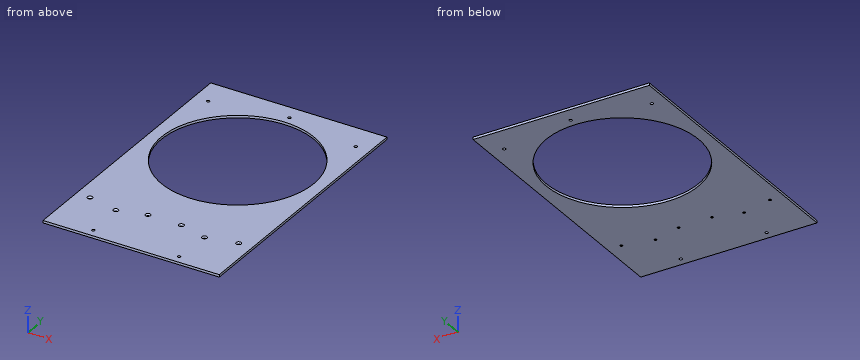
```python
from build123d import *

# Parameters (mm, degrees)
SKETCH1_W                                     = 469.9
SKETCH1_H                                     = 2413
SKETCH1_R                                     = 203.2
BOSS_EXTRUDE1_DEPTH                           = 6.35
CSK_FOR_1_4_FLAT_HEAD_SOCKET_CAP_SCR_2_COUNT  = 2
CSK_FOR_1_4_FLAT_HEAD_SOCKET_CAP_SCR_2_PITCH  = 76.2
CSK_FOR_1_4_FLAT_HEAD_SOCKET_CAP_SCR_3_COUNT  = 2
CSK_FOR_1_4_FLAT_HEAD_SOCKET_CAP_SCR_3_PITCH  = 89.142542345
CSK_FOR_1_4_FLAT_HEAD_SOCKET_CAP_SCR_4_COUNT  = 2
CSK_FOR_1_4_FLAT_HEAD_SOCKET_CAP_SCR_4_PITCH  = 163.936718394
CSK_FOR_1_4_FLAT_HEAD_SOCKET_CAP_SCR_5_COUNT  = 2
CSK_FOR_1_4_FLAT_HEAD_SOCKET_CAP_SCR_5_PITCH  = 711.2
CSK_FOR_1_4_FLAT_HEAD_SOCKET_CAP_SCR_6_COUNT  = 2
CSK_FOR_1_4_FLAT_HEAD_SOCKET_CAP_SCR_6_PITCH  = 695.384275934
CSK_FOR_1_4_FLAT_HEAD_SOCKET_CAP_SCR_7_COUNT  = 2
CSK_FOR_1_4_FLAT_HEAD_SOCKET_CAP_SCR_7_PITCH  = 716.764837904
CSK_FOR_1_4_FLAT_HEAD_SOCKET_CAP_SCR_8_COUNT  = 2
CSK_FOR_1_4_FLAT_HEAD_SOCKET_CAP_SCR_8_PITCH  = 710.371803251
CSK_FOR_1_4_FLAT_HEAD_SOCKET_CAP_SCR_9_COUNT  = 2
CSK_FOR_1_4_FLAT_HEAD_SOCKET_CAP_SCR_9_PITCH  = 1422.4
CSK_FOR_1_4_FLAT_HEAD_SOCKET_CAP_SCR_10_COUNT = 2
CSK_FOR_1_4_FLAT_HEAD_SOCKET_CAP_SCR_10_PITCH = 1404.60778242
CSK_FOR_1_4_FLAT_HEAD_SOCKET_CAP_SCR_11_COUNT = 2
CSK_FOR_1_4_FLAT_HEAD_SOCKET_CAP_SCR_11_PITCH = 1425.190567207
CSK_FOR_1_4_FLAT_HEAD_SOCKET_CAP_SCR_12_COUNT = 2
CSK_FOR_1_4_FLAT_HEAD_SOCKET_CAP_SCR_12_PITCH = 1412.087755797
CSK_FOR_1_4_FLAT_HEAD_SOCKET_CAP_SCR_13_COUNT = 2
CSK_FOR_1_4_FLAT_HEAD_SOCKET_CAP_SCR_13_PITCH = 153.55813077
CSK_FOR_1_4_FLAT_HEAD_SOCKET_CAP_SCR_14_COUNT = 2
CSK_FOR_1_4_FLAT_HEAD_SOCKET_CAP_SCR_14_PITCH = 242.697219812
CSK_FOR_1_4_FLAT_HEAD_SOCKET_CAP_SCR_15_COUNT = 2
CSK_FOR_1_4_FLAT_HEAD_SOCKET_CAP_SCR_15_PITCH = 749.86024568
CSK_FOR_1_4_FLAT_HEAD_SOCKET_CAP_SCR_16_COUNT = 2
CSK_FOR_1_4_FLAT_HEAD_SOCKET_CAP_SCR_16_PITCH = 1441.280581843
CSK_FOR_1_4_FLAT_HEAD_SOCKET_CAP_SCR_17_COUNT = 2
CSK_FOR_1_4_FLAT_HEAD_SOCKET_CAP_SCR_17_PITCH = 1428.974413563
CSK_FOR_1_4_FLAT_HEAD_SOCKET_CAP_SCR_18_COUNT = 2
CSK_FOR_1_4_FLAT_HEAD_SOCKET_CAP_SCR_18_PITCH = 725.925992834
F_5_16_0_3125_DIAMETER_HOLE1_D                = 7.9375
SKETCH6_W                                     = 469.9
SKETCH6_H                                     = 1654.81
CUT_EXTRUDE1_DEPTH                            = 7.35
SKETCH7_W                                     = 469.9
SKETCH7_H                                     = 27.94
CUT_EXTRUDE2_DEPTH                            = 7.35


with BuildPart() as part:
    # Sketch1 → Boss-Extrude1 (new body)
    with BuildSketch(Plane.XY):
        with Locations((0, 1206.5)):
            Rectangle(SKETCH1_W, SKETCH1_H)
        with Locations((0, 695.96)):
            Circle(SKETCH1_R, mode=Mode.SUBTRACT)
        with Locations((0, 1407.16)):
            Circle(SKETCH1_R, mode=Mode.SUBTRACT)
        with Locations((0, 2118.36)):
            Circle(SKETCH1_R, mode=Mode.SUBTRACT)
    extrude(amount=BOSS_EXTRUDE1_DEPTH)

    # Sketch3 → CSK for 1/4 Flat Head Socket Cap Screw1 (revolve, cut)
    with BuildSketch(Plane(origin=(44.571271172, 378.545152647, 6.35), x_dir=(0, -1, 0), z_dir=(1, 0, 0))):
        Polygon((0, 0), (0, 6.35), (3.3782, 6.35), (3.3782, 3.871564875), (6.7437, 0), align=None)
    csk_for_1_4_flat_head_socket_cap_screw1 = revolve(axis=Axis((44.571271172, 378.545152647, 12.7), (0, 0, -1)), mode=Mode.SUBTRACT)

    # CSK for 1_4 Flat Head Socket Cap Scr 2: CSK for 1/4 Flat Head Socket Cap Screw1 ×2
    with Locations(*[Vector(0.965925826, -0.258819045, 0) * (i * CSK_FOR_1_4_FLAT_HEAD_SOCKET_CAP_SCR_2_PITCH) for i in range(1, CSK_FOR_1_4_FLAT_HEAD_SOCKET_CAP_SCR_2_COUNT)]):
        add(csk_for_1_4_flat_head_socket_cap_screw1, mode=Mode.SUBTRACT)

    # CSK for 1_4 Flat Head Socket Cap Scr 3: CSK for 1/4 Flat Head Socket Cap Screw1 ×2
    with Locations(*[(-i * CSK_FOR_1_4_FLAT_HEAD_SOCKET_CAP_SCR_3_PITCH, 0, 0) for i in range(1, CSK_FOR_1_4_FLAT_HEAD_SOCKET_CAP_SCR_3_COUNT)]):
        add(csk_for_1_4_flat_head_socket_cap_screw1, mode=Mode.SUBTRACT)

    # CSK for 1_4 Flat Head Socket Cap Scr 4: CSK for 1/4 Flat Head Socket Cap Screw1 ×2
    with Locations(*[Vector(-0.99273727, -0.120302586, 0) * (i * CSK_FOR_1_4_FLAT_HEAD_SOCKET_CAP_SCR_4_PITCH) for i in range(1, CSK_FOR_1_4_FLAT_HEAD_SOCKET_CAP_SCR_4_COUNT)]):
        add(csk_for_1_4_flat_head_socket_cap_screw1, mode=Mode.SUBTRACT)

    # CSK for 1_4 Flat Head Socket Cap Scr 5: CSK for 1/4 Flat Head Socket Cap Screw1 ×2
    with Locations(*[(0, i * CSK_FOR_1_4_FLAT_HEAD_SOCKET_CAP_SCR_5_PITCH, 0) for i in range(1, CSK_FOR_1_4_FLAT_HEAD_SOCKET_CAP_SCR_5_COUNT)]):
        add(csk_for_1_4_flat_head_socket_cap_screw1, mode=Mode.SUBTRACT)

    # CSK for 1_4 Flat Head Socket Cap Scr 6: CSK for 1/4 Flat Head Socket Cap Screw1 ×2
    with Locations(*[Vector(0.105845862, 0.994382549, 0) * (i * CSK_FOR_1_4_FLAT_HEAD_SOCKET_CAP_SCR_6_PITCH) for i in range(1, CSK_FOR_1_4_FLAT_HEAD_SOCKET_CAP_SCR_6_COUNT)]):
        add(csk_for_1_4_flat_head_socket_cap_screw1, mode=Mode.SUBTRACT)

    # CSK for 1_4 Flat Head Socket Cap Scr 7: CSK for 1/4 Flat Head Socket Cap Screw1 ×2
    with Locations(*[Vector(-0.124367907, 0.992236173, 0) * (i * CSK_FOR_1_4_FLAT_HEAD_SOCKET_CAP_SCR_7_PITCH) for i in range(1, CSK_FOR_1_4_FLAT_HEAD_SOCKET_CAP_SCR_7_COUNT)]):
        add(csk_for_1_4_flat_head_socket_cap_screw1, mode=Mode.SUBTRACT)

    # CSK for 1_4 Flat Head Socket Cap Scr 8: CSK for 1/4 Flat Head Socket Cap Screw1 ×2
    with Locations(*[Vector(-0.229099874, 0.973402922, 0) * (i * CSK_FOR_1_4_FLAT_HEAD_SOCKET_CAP_SCR_8_PITCH) for i in range(1, CSK_FOR_1_4_FLAT_HEAD_SOCKET_CAP_SCR_8_COUNT)]):
        add(csk_for_1_4_flat_head_socket_cap_screw1, mode=Mode.SUBTRACT)

    # CSK for 1_4 Flat Head Socket Cap Scr 9: CSK for 1/4 Flat Head Socket Cap Screw1 ×2
    with Locations(*[(0, i * CSK_FOR_1_4_FLAT_HEAD_SOCKET_CAP_SCR_9_PITCH, 0) for i in range(1, CSK_FOR_1_4_FLAT_HEAD_SOCKET_CAP_SCR_9_COUNT)]):
        add(csk_for_1_4_flat_head_socket_cap_screw1, mode=Mode.SUBTRACT)

    # CSK for 1_4 Flat Head Socket Cap Scr 10: CSK for 1/4 Flat Head Socket Cap Screw1 ×2
    with Locations(*[Vector(0.052401495, 0.998626098, 0) * (i * CSK_FOR_1_4_FLAT_HEAD_SOCKET_CAP_SCR_10_PITCH) for i in range(1, CSK_FOR_1_4_FLAT_HEAD_SOCKET_CAP_SCR_10_COUNT)]):
        add(csk_for_1_4_flat_head_socket_cap_screw1, mode=Mode.SUBTRACT)

    # CSK for 1_4 Flat Head Socket Cap Scr 11: CSK for 1/4 Flat Head Socket Cap Screw1 ×2
    with Locations(*[Vector(-0.062547805, 0.998041969, 0) * (i * CSK_FOR_1_4_FLAT_HEAD_SOCKET_CAP_SCR_11_PITCH) for i in range(1, CSK_FOR_1_4_FLAT_HEAD_SOCKET_CAP_SCR_11_COUNT)]):
        add(csk_for_1_4_flat_head_socket_cap_screw1, mode=Mode.SUBTRACT)

    # CSK for 1_4 Flat Head Socket Cap Scr 12: CSK for 1/4 Flat Head Socket Cap Screw1 ×2
    with Locations(*[Vector(-0.115252108, 0.993336273, 0) * (i * CSK_FOR_1_4_FLAT_HEAD_SOCKET_CAP_SCR_12_PITCH) for i in range(1, CSK_FOR_1_4_FLAT_HEAD_SOCKET_CAP_SCR_12_COUNT)]):
        add(csk_for_1_4_flat_head_socket_cap_screw1, mode=Mode.SUBTRACT)

    # CSK for 1_4 Flat Head Socket Cap Scr 13: CSK for 1/4 Flat Head Socket Cap Screw1 ×2
    with Locations(*[Vector(0.999938773, -0.011065747, 0) * (i * CSK_FOR_1_4_FLAT_HEAD_SOCKET_CAP_SCR_13_PITCH) for i in range(1, CSK_FOR_1_4_FLAT_HEAD_SOCKET_CAP_SCR_13_COUNT)]):
        add(csk_for_1_4_flat_head_socket_cap_screw1, mode=Mode.SUBTRACT)

    # CSK for 1_4 Flat Head Socket Cap Scr 14: CSK for 1/4 Flat Head Socket Cap Screw1 ×2
    with Locations(*[Vector(-0.999975489, -0.007001462, 0) * (i * CSK_FOR_1_4_FLAT_HEAD_SOCKET_CAP_SCR_14_PITCH) for i in range(1, CSK_FOR_1_4_FLAT_HEAD_SOCKET_CAP_SCR_14_COUNT)]):
        add(csk_for_1_4_flat_head_socket_cap_screw1, mode=Mode.SUBTRACT)

    # CSK for 1_4 Flat Head Socket Cap Scr 15: CSK for 1/4 Flat Head Socket Cap Screw1 ×2
    with Locations(*[Vector(-0.32364867, 0.946177329, 0) * (i * CSK_FOR_1_4_FLAT_HEAD_SOCKET_CAP_SCR_15_PITCH) for i in range(1, CSK_FOR_1_4_FLAT_HEAD_SOCKET_CAP_SCR_15_COUNT)]):
        add(csk_for_1_4_flat_head_socket_cap_screw1, mode=Mode.SUBTRACT)

    # CSK for 1_4 Flat Head Socket Cap Scr 16: CSK for 1/4 Flat Head Socket Cap Screw1 ×2
    with Locations(*[Vector(-0.168385861, 0.985721158, 0) * (i * CSK_FOR_1_4_FLAT_HEAD_SOCKET_CAP_SCR_16_PITCH) for i in range(1, CSK_FOR_1_4_FLAT_HEAD_SOCKET_CAP_SCR_16_COUNT)]):
        add(csk_for_1_4_flat_head_socket_cap_screw1, mode=Mode.SUBTRACT)

    # CSK for 1_4 Flat Head Socket Cap Scr 17: CSK for 1/4 Flat Head Socket Cap Screw1 ×2
    with Locations(*[Vector(0.107453799, 0.994210079, 0) * (i * CSK_FOR_1_4_FLAT_HEAD_SOCKET_CAP_SCR_17_PITCH) for i in range(1, CSK_FOR_1_4_FLAT_HEAD_SOCKET_CAP_SCR_17_COUNT)]):
        add(csk_for_1_4_flat_head_socket_cap_screw1, mode=Mode.SUBTRACT)

    # CSK for 1_4 Flat Head Socket Cap Scr 18: CSK for 1/4 Flat Head Socket Cap Screw1 ×2
    with Locations(*[Vector(0.211521189, 0.977373412, 0) * (i * CSK_FOR_1_4_FLAT_HEAD_SOCKET_CAP_SCR_18_PITCH) for i in range(1, CSK_FOR_1_4_FLAT_HEAD_SOCKET_CAP_SCR_18_COUNT)]):
        add(csk_for_1_4_flat_head_socket_cap_screw1, mode=Mode.SUBTRACT)

    # 5/16 (0.3125) Diameter Hole1 (through all)
    with Locations(Plane.XY.offset(6.35)):
        with Locations((-114.3, 254.635), (-114.3, 210.185), (-196.85, 177.8), (196.85, 177.8), (114.3, 210.185), (114.3, 254.635), (-114.3, 965.835), (-114.3, 921.385), (-196.85, 889), (196.85, 889), (114.3, 921.385), (114.3, 965.835), (-114.3, 1677.035), (-114.3, 1632.585), (-196.85, 1600.2), (196.85, 1600.2), (114.3, 1632.585), (114.3, 1677.035), (-196.85, 2311.4), (196.85, 2311.4), (0, 2343.785)):
            Hole(F_5_16_0_3125_DIAMETER_HOLE1_D / 2)

    # Sketch6 → Cut-Extrude1 (cut, through all)
    with BuildSketch(Plane.XY.offset(6.35)):
        with Locations((0, 827.405)):
            Rectangle(SKETCH6_W, SKETCH6_H)
    extrude(amount=-CUT_EXTRUDE1_DEPTH, mode=Mode.SUBTRACT)

    # Sketch7 → Cut-Extrude2 (cut, through all)
    with BuildSketch(Plane.XY.offset(6.35)):
        with Locations((0, 2399.03)):
            Rectangle(SKETCH7_W, SKETCH7_H)
    extrude(amount=-CUT_EXTRUDE2_DEPTH, mode=Mode.SUBTRACT)


solid = part.part
```
CAD build for the part. Positions are in the model's coordinates, mm. Give positions to 0.01 mm unless a question says otherwise; leave off trailing zeros. Order: outer loops, then holes, each group sorted by start corner. A loop starts at its lowest first (then second) coordinate and runs counter-clockwise, first axis right, second up.
(1) Saw through at B-B, the plane x = -25.5. Give the cut face in (y, z), then the cut area to 3 significant figures.
(2) Drill centre lines: L1, parallel to Y at x = 0, z = 3.75; L2, parallel to X at y = 1776, z = 6.25; L3, parallel to Y at x = 6, z = 2.75. Where is each one in solid material? Low to high.
(3) Flat gauge pin, fed straight in: pin 1 (12.5 mm diameter, centred on x = -114.3, y = 1677.035, fed in from +Z). Where does the tip first touch, or does it go through?
(4) Saw through at C-C, the plane z = 4.25. State how many separate pieces and enclosed holes the cut face has, then the cut area to 3 significant figures.
(5) Saw through at A-A, the plane y = 2052. Give the cut face in (x, z).
Results found:
1. outline: (1654.81, 0) - (1916.77, 0) - (1916.77, 6.35) - (1654.81, 6.35) - close; (2319.95, 0) - (2385.06, 0) - (2385.06, 6.35) - (2319.95, 6.35) - close
1. area: 2,080 mm2
2. L1: y = 1654.81 to 1915.16, 2321.56 to 2339.82, 2347.75 to 2385.06
2. L2: x = -234.95 to -122.3, -114.05 to 114.05, 122.3 to 234.95
2. L3: y = 1654.81 to 1915.25, 2321.47 to 2385.06
3. pin 1: stops at z = 6.35
4. separate pieces: 1
4. enclosed holes: 12
4. area: 213,000 mm2
5. outline: (-234.95, 0) - (-192.06, 0) - (-192.06, 6.35) - (-234.95, 6.35) - close; (192.06, 0) - (234.95, 0) - (234.95, 6.35) - (192.06, 6.35) - close
